The listing builds one solid part. Answer for the finished solid, in the listing's coordinates (mm). A direction names the side the tool comes from. Round coordinates to 2 decimals unless told otherwise and drop trailing zeros. Order: outer loops, then holes, each group sorted by start corner. A loop starts at its lowest first (then second) coordinate and runs counter-clockwise, first axis right, second up. Notation, with made-up numbers: (29.5, 7) - (65.5, 7) arc R22 ccw to (65.5, 36) - close; hole circle Ø1 at (33.5, 85). An arc over 180 degrees is marked (long way). One line per item, written item: value. Start each with the question number.
1. For a pull along X with two mould halves and no side action, classify faces 1 (the flat face through (12.5, 26, 22)), 2 (the flat face through (-15, 38, 37)), 3 (the flat face through (-17.5, 21, 21)) as released by +X, released by -X, zero draft, split by the parting line, or undercut.
2. Straight lines are drawn through the part: line 1 (Z direction, x = 0, y = 5); line 2 (X direction, y = 6, z = 50); line 3 (X direction, y = 37, z = 8.5). For each, find the intervals that lie inside material, in ascending order.
3. A tool of negligible diameter and unlimited length cuts with its end or side. For faces 4 (the flat face through (0, 10, 35)), 5 (the flat face through (0, 37, 0)), from which of +Z, -Z, +X, -X, +Y, -Y can it reach the whole face along a straight path? Write none if from no direction.
4. Flat-ended cylindrical pins translate along their axes: P1, Ø4, axis at x = -12, y = 44, coming from the +Z side; P2, Ø1, axis at x = -4, z = 27.5, coming from the +Y side; P3, Ø8, axis at x = -6, y = 38, coming from the +Z side; P4, Ø4, axis at x = 0, z = 50, coming from the +Y side. Find the tip coordinate at first contact, or state that the pin passes through.
5. Section C-C, the plane y = 28 is taken. Give the vertices of the cut face in (x, z).
6. Section D-D, the plane z = 58 is taken. Give the vertices of the cut face in (x, y), then the cut area to 3 significant figures.
7. Section A-A, the plane x = 0 is taken. Give the vertices of the cut face in (y, z).
8. Section B-B, the plane z = 20 is taken. Give the vertices of the cut face in (x, y).
from build123d import *

# Parameters (mm, degrees)
BOSS_EXTRUDE1_DEPTH   = 17.5
CUT_EXTRUDE1_START    = 10
SKETCH2_W             = 25
SKETCH2_H             = 70
CUT_EXTRUDE1_DEPTH    = 98.5
F_6_0MM_DOWEL_HOLE1_D = 6.5


with BuildPart() as part:
    # Sketch1 → Boss-Extrude1 (new, symmetric)
    with BuildSketch(Plane(origin=(0, 0, 0), x_dir=(0, 0, -1), z_dir=(1, 0, 0))):
        Polygon((0, 0), (0, 75), (-75, 0), align=None)
    extrude(amount=BOSS_EXTRUDE1_DEPTH, both=True)

    # Sketch2 → Cut-Extrude1 (cut, through all)
    with BuildSketch(Plane(origin=(0, 0, 0), x_dir=(1, 0, 0), z_dir=(0, 1, 0)).offset(CUT_EXTRUDE1_START)):
        with Locations((0, -40)):
            Rectangle(SKETCH2_W, SKETCH2_H)
    extrude(amount=CUT_EXTRUDE1_DEPTH, mode=Mode.SUBTRACT)

    # Ø6.0mm Dowel Hole1 (through all)
    with Locations(Plane(origin=(0, 10, 0), x_dir=(1, 0, 0), z_dir=(0, 1, 0))):
        with Locations((0, -20), (0, -50)):
            Hole(F_6_0MM_DOWEL_HOLE1_D / 2)


solid = part.part
Answer list:
1. face 1: undercut
1. face 2: zero draft
1. face 3: released by -X
2. line 1: z = 0 to 16.75, 23.25 to 46.75, 53.25 to 70
2. line 2: x = -17.5 to -3.25, 3.25 to 17.5
2. line 3: x = -17.5 to -12.5, 12.5 to 17.5
3. face 4: +Z, +Y
3. face 5: -Z, +X, -X, +Y, -Y
4. P1: stops at z = 32.94
4. P2: stops at y = 10
4. P3: stops at z = 5
4. P4: passes through
5. outline: (-17.5, 0) - (17.5, 0) - (17.5, 47) - (12.5, 47) - (12.5, 5) - (-12.5, 5) - (-12.5, 47) - (-17.5, 47) - close
6. outline: (-17.5, 0) - (17.5, 0) - (17.5, 17) - (12.5, 17) - (12.5, 10) - (-12.5, 10) - (-12.5, 17) - (-17.5, 17) - close
6. area: 420 mm²
7. outline: (0, 0) - (75, 0) - (70, 5) - (10, 5) - (10, 16.75) - (0, 16.75) - close; (0, 23.25) - (10, 23.25) - (10, 46.75) - (0, 46.75) - close; (0, 53.25) - (10, 53.25) - (10, 65) - (0, 75) - close
8. outline: (-17.5, 0) - (-3.25, 0) - (-3.25, 10) - (-12.5, 10) - (-12.5, 55) - (-17.5, 55) - close; (3.25, 0) - (17.5, 0) - (17.5, 55) - (12.5, 55) - (12.5, 10) - (3.25, 10) - close
